Can you work these out from the model? Positions are in its coordinate system, mm. A direction names the side the tool comes from. Coordinates: 2 decimals unless noted, no trailing zeros. Write each loop counter-clockwise with the first axis right and the second up, starting at its lowest first coordinate (ties: lowest second). Pieces come first, ordered by that corner, then holes. Notation, with made-up numbers: (86.5, -4) - (127.5, -4) arc R35 cw to (127.5, 28) - close; hole circle Ø7 at (3, 57). An arc over 180 degrees is marked (long way). Use one line per item in the form item = value. Start each with the question number.
(1) On a 3-axis mill with a long thin cutter (end or side, diameter ignored), from which of +Z, -Z, +X, -X, +Y, -Y can I reach the whole of each face in a straight line? I mean faces 1 (the face through (2.731, 4.554, 2.535)), 2 (the face through (3.53, -9.486, 2.535)). Say none if no direction works.
(2) If we section it at C-C on x = 16: Please give me the cut outline in (y, z), then the cut area to 3 significant figures.
(3) Thinking about a two-plate mould opening in Y: for faces 3 (the face through (2.55, 10, 2)), 4 (the face through (7.1, -8.4, 2.5)), 5 (the face through (5.05, 0.06, 2.46)), 6 (the face through (54, 60.75, 2)), which applies, pulls with the +Y half, pulls with the -Y half, needs draft (parallel to the pull), parting line crosses it, or undercut?
(4) For pin 1 Ø2 at (y, z) = (43.5, 3) entering from -X; pin 2 Ø12 at (x, y) = (21, 6) entering from +Z; pin 3 Ø1.5 at (x, z) = (43.5, 1.5) entering from -Y; pin 4 Ø3 at (x, z) = (17.5, 2.5) entering from -Y, each with a flat end and sliding along its axis, tell me the tip position at first contact or that it passes through.
(5) If we section it at B-B on y = 35: Please give me the cut outline in (x, z), then the cut area to 3 significant figures.
(6) If I drill on probe 1 along Y at (x, z) = (18.5, 4.5); probe 2 along X at (y, z) = (32, 4.8); probe 3 along Y at (x, z) = (25, 1), over which ranges is the centre line in solid material (lowest first)? Write a range as from..to.
(7) If we section it at A-A on z = 3.95: Please give me the cut outline in (x, y).
Autodesk Inventor part; units mm, degrees
ref_plane "YZ Plane" through (0, 0, 0) normal (1, 0, 0) x (0, 1, 0)
ref_plane "XZ Plane" through (0, 0, 0) normal (0, 1, 0) x (-1, 0, 0)
ref_plane "XY Plane" through (0, 0, 0) normal (0, 0, 1) x (1, 0, 0)
sketch "スケッチ1" plane through (0, 0, 0) normal (0, 0, 1) x (1, 0, 0)
  circle A0 centre (0, 0) radius 11 construction
  circle A1 centre (0, 8.5) radius 1.35
  circle A2 centre (0, 8.5) radius 2.5 construction
  circle A3 centre (0, 0) radius 5.05 construction
  circle A4 centre (0, -8.5) radius 1.35
  line L0 (48.7145, 60.75) -> (2.55, 14.5855)
  line L1 (0, 0) -> (0, 48.2635) construction
  line L2 (60.75, 60.75) -> (0, 0) construction
  line L3 (48.7145, 60.75) -> (60.75, 60.75)
  line L4 (60.75, 60.75) -> (60.75, 55.75)
  arc A5 (2.55, -10.7004) -> (8.4522, -7.0399) centre (0, 0) ccw
  line L5 (60.75, 55.75) -> (8.4522, -7.0399)
  circle A6 centre (0, 0) radius 8.5 construction
  circle A7 centre (8.5, 0) radius 1.35
  line L6 (2.55, 14.5855) -> (2.55, 4.3589)
  arc A8 (2.55, -4.3589) -> (2.55, 4.3589) centre (0, 0) ccw
  line L7 (2.55, -4.3589) -> (2.55, -10.7004)
  dimension "d3" = 10.1
  dimension "d0" = 2.7
  dimension "d1" = 8.5
  dimension "d2" = 5
  dimension "d6" = 360
  dimension "d11" = 45
  dimension "d13" = 60.75
  dimension "d17" = 5
  dimension "d18" = 2.55
extrude "押し出し1" add sketch "スケッチ1" along normal blind 5 contours L3 L4 L5 A5 L7 A8 L6 L0
fillet "フィレット1" radius 2 7 edges at (2.55, -10.7004, 2.5) (2.55, -4.3589, 2.5) (2.55, 14.5855, 2.5) (60.75, 60.75, 2.5) (60.75, 55.75, 2.5) (48.7145, 60.75, 2.5) (2.55, 4.3589, 2.5)
sketch "スケッチ3" plane through (0, 0, 0) normal (0, 0, -1) x (-1, 0, 0)
  circle A0 centre (-8.5, 0) radius 1.35
  circle A1 centre (-8.5, 0) radius 1.35
  point P0 (0, 0)
extrude "押し出し3" add sketch "スケッチ3" against normal up to surface (5 mm away) from surface at 0
ref_plane "作業平面1" through (0, 0, 4) normal (0, 0, -1) x (-1, 0, 0)
sketch "スケッチ4" plane through (0, 0, 4) normal (0, 0, -1) x (-1, 0, 0)
  point P0 (0, 0)
properties part number "頭_サブフレーム_1_1" material "アセタール樹脂、黒"
Reported:
q1.face_1 = +Z, -Z, -X
q1.face_2 = +Z, -Z, -Y
q2.outline = (2.02, 0) - (28.04, 0) - (28.04, 5) - (2.02, 5) - close
q2.area = 130 mm2
q3.face_3 = needs draft
q3.face_4 = pulls with the -Y half
q3.face_5 = undercut
q3.face_6 = pulls with the +Y half
q4.pin_1 = 30.46
q4.pin_2 = 5
q4.pin_3 = 34.14
q4.pin_4 = 2.02
q5.outline = (22.96, 0) - (43.47, 0) - (43.47, 5) - (22.96, 5) - close
q5.area = 103 mm2
q6.probe_1 = 5.02..30.54
q6.probe_2 = 19.96..40.97
q6.probe_3 = 12.83..37.04
q7.outline = (2.55, -7.77) arc R2 ccw to (5.56, -9.49) arc R11 ccw to (8.45, -7.04) - (60.29, 55.19) arc R2 ccw to (60.75, 56.47) - (60.75, 58.75) arc R2 ccw to (58.75, 60.75) - (49.54, 60.75) arc R2 ccw to (48.13, 60.16) - (3.14, 15.17) arc R2 ccw to (2.55, 13.76) - (2.55, 5.39) arc R2 ccw to (3.26, 3.86) arc R5.05 cw to (3.26, -3.86) arc R2 ccw to (2.55, -5.39) - close
